Geometry check sheet. Reference: drawing and pictorial views, mm from the part's lowest x, y, z. A direction names the side the tool comes from. Round coordinates to 2 decimals unless told otherwise and drop trailing zeros. Write each loop counter-clockwise with the first axis right and the second up, starting at its lowest first coordinate (ties: lowest second). Pieces come first, ordered by that corner, then holes. Notation, with made-up numbers: M 71.25,35.25 L 95.25,35.25 A26 cw 95.25,67.25 Z; hole C 11.25,85.25 d4. An arc over 180 degrees is marked long. Answer in a Markdown table with one row per item. Add a question column.
1. Sectioned sample at D-D on x = 7.25. Record the cut outline in (y, z).
2. Go/stop test with a flat-tipped pin: pin 1 Ø5.5 at (x, y) = (5, 5) entering from -Z. Record where the tip stops, or that it passes through.
3. Set-up check for the marked faces 4 and 5: record each of +Z, -Z, +X, -X, +Y, -Y from which the full face is reachable in a straight line by a thin tool's end or side.
4. Sectioned sample at C-C on y = 6.5. Record the cut outline in (x, z).
5. Draft check along Y on the marked faces 1, 2 and 3. Enter one of: pulls with the +Y half, pulls with the -Y half, needs draft (parallel to the pull), parting line crosses it, or undercut.
6. Sectioned sample at B-B on x = 5. Record the cut outline in (y, z).
7. Material ranges on probe 1 along X at (y, z) = (4.25, 5); probe 2 along Y at (x, z) = (7, 2.5) (1 decimal); probe 3 along Y at (x, z) = (5, 4.55), recorded low to high.
8. Sectioned sample at A-A on z = 4.75. Record the cut outline in (x, y).
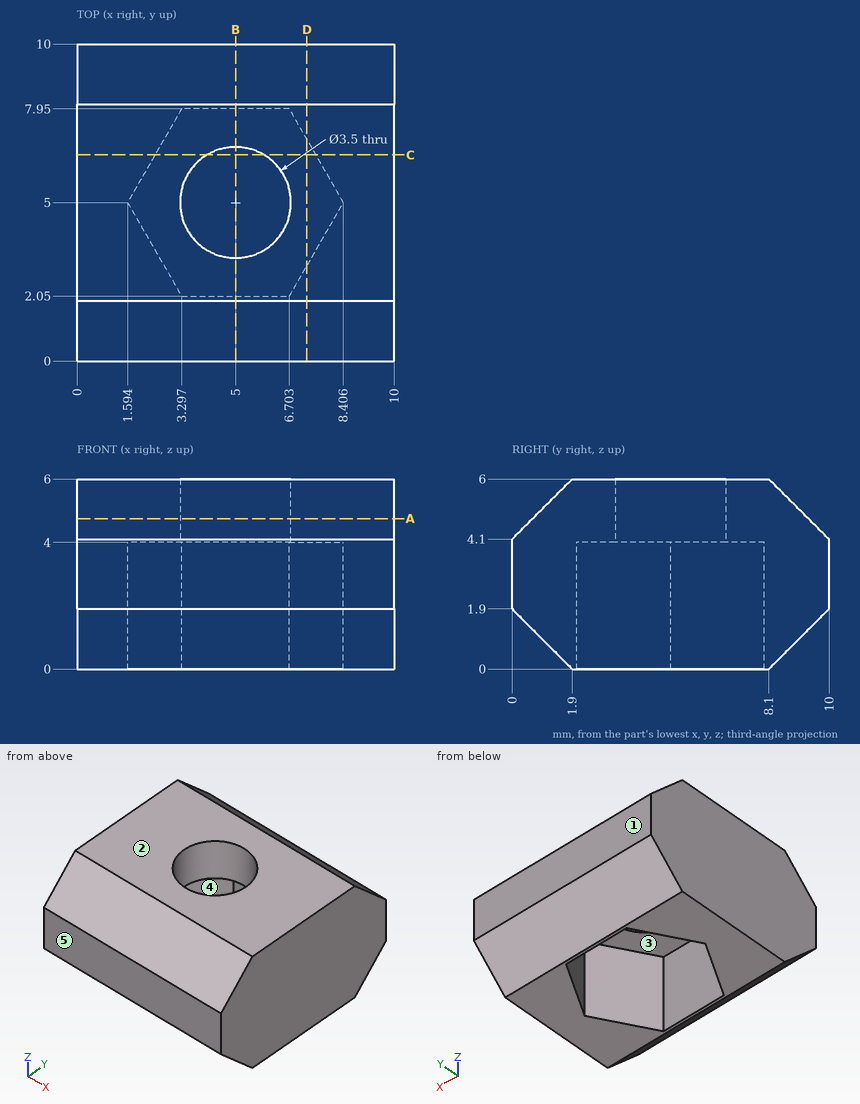
Geometry check:
| question | item | result |
|---|---|---|
| 1 | outline | M 0,1.9 L 1.9,0 L 3,0 L 3,4 L 7,4 L 7,0 L 8.1,0 L 10,1.9 L 10,4.1 L 8.1,6 L 1.9,6 L 0,4.1 Z |
| 2 | pin 1 | stops at z = 4 |
| 3 | face 4 | -Z |
| 3 | face 5 | +Z, -Z, +X, -X, -Y |
| 4 | outline | M 0,0 L 2.46,0 L 2.46,4 L 4.1,4 L 4.1,6 L 0,6 Z; M 5.9,4 L 7.54,4 L 7.54,0 L 10,0 L 10,6 L 5.9,6 Z |
| 5 | face 1 | pulls with the +Y half |
| 5 | face 2 | needs draft |
| 5 | face 3 | undercut |
| 6 | outline | M 0,1.9 L 1.9,0 L 2.05,0 L 2.05,4 L 3.25,4 L 3.25,6 L 1.9,6 L 0,4.1 Z; M 6.75,4 L 7.95,4 L 7.95,0 L 8.1,0 L 10,1.9 L 10,4.1 L 8.1,6 L 6.75,6 Z |
| 7 | probe 1 | x = 0 to 3.42, 6.58 to 10 |
| 7 | probe 2 | y = 0 to 2.6, 7.4 to 10 |
| 7 | probe 3 | y = 0.45 to 3.25, 6.75 to 9.55 |
| 8 | outline | M 0,0.65 L 10,0.65 L 10,9.35 L 0,9.35 Z; hole C 5,5 d3.5 |
